Geometry: final body of the model. Coordinates: model frame, mm. Face numbers are marked on the shaded views. A direction names the side the tool comes from. Round coordinates to 2 decimals unless told otherwise and drop trailing zeros. Order: outer loops, then holes, each group sorted by start corner. A loop starts at its lowest first (then second) coordinate and runs counter-clockwise, first axis right, second up. Notation, with made-up numbers: M -26,14 L 8,14 A20 cw 8,52 Z; hole C -30.75,49.5 d8. An arc over 180 degrees is marked long. Return JSON: item names as keys, results as strings. Group by question number.
Q1. Contact query for flat-ended pins moving along their axis: pin 1 (3 mm diameter, centred on x = -41, z = 4.5, fed in from +Y); pin 2 (1.3 mm diameter, centred on y = 27, z = 6, fed in from +X). Output: stop coordinate, or through.
Q2. Ray query, probe 1 along X at (y, z) = (28, 4.5); probe 2 along X at (y, z) = (35.5, 2); probe 3 along X at (y, z) = (26.75, 7.75). Return the intervals inside material, ascending.
Q3. Cut plane B-B on y = 32. Output: boundary loops of the cut face in (x, z).
Q4. Access query for the marked faces 5, 6 and 7. Directions: +Z, -Z, +X, -X, +Y, -Y. A direction counts if a zero-diameter tool reaches every point of the face in a straight line with its end or side. Return the directions, or none.
Q5. Cut plane A-A on z = 5. Output: boundary loops of the cut face in (x, y).
Q6. Cut plane C-C on y = 20.5. Output: boundary loops of the cut face in (x, z), and give its area (3 significant figures).
Q7. Mould query, pull axis X, two halves, no side actions, for the marked faces 1, 2, 3 and 4. Classes: released by +X, released by -X, zero draft, split by the parting line, or undercut.
Q8. Cut plane D-D on x = -45. Output: boundary loops of the cut face in (y, z).
```python
from build123d import *

# Parameters (mm, degrees)
F0_W     = 20
F0_H     = 14.121413
F1_DEPTH = 10
F2_R     = 2.65
F3_DEPTH = 9.901
F5_DEPTH = 10


with BuildPart() as f1:
    # F0 (on Top) → F1 (new body)
    with BuildSketch(Plane.XY):
        with Locations((-41.761377, 22.08462)):
            Rectangle(F0_W, F0_H)
        with BuildLine():
            ThreePointArc((-25.361377, 20.023914), (-26.738101, 21.169687), (-25.861377, 22.731583))
            Line((-25.861377, 22.731583), (-25.861377, 26.782085))
            Line((-25.861377, 26.782085), (-25.861377, 27.804352))
            Line((-25.861377, 27.804352), (-25.861377, 36.782085))
            Line((-25.861377, 36.782085), (-28.861377, 36.782085))
            Line((-28.861377, 36.782085), (-28.861377, 29.145327))
            Line((-28.861377, 29.145327), (-31.761377, 29.145327))
            Line((-31.761377, 29.145327), (-31.761377, 15.023914))
            Line((-31.761377, 15.023914), (-25.361377, 15.023914))
            Line((-25.361377, 15.023914), (-25.361377, 20.023914))
        make_face()
        with BuildLine():
            ThreePointArc((-24.861377, 22.731583), (-23.984653, 21.169687), (-25.361377, 20.023914))
            Line((-25.361377, 20.023914), (-25.361377, 15.023914))
            ThreePointArc((-25.361377, 15.023914), (-19.227361, 19.59803), (-21.861377, 26.782085))
            Line((-21.861377, 26.782085), (-21.861377, 36.782085))
            Line((-21.861377, 36.782085), (-24.861377, 36.782085))
            Line((-24.861377, 36.782085), (-24.861377, 27.804352))
            Line((-24.861377, 27.804352), (-24.861377, 26.782085))
            Line((-24.861377, 26.782085), (-24.861377, 22.731583))
        make_face()
    extrude(amount=F1_DEPTH)

    # F2 (on face) → F3 (cut, through all)
    with BuildSketch(Plane(origin=(-28.861377, 0, 0), x_dir=(0, -1, 0), z_dir=(-1, 0, 0))):
        with Locations((-32.963706, 5)):
            Circle(F2_R)
    extrude(amount=-F3_DEPTH, mode=Mode.SUBTRACT)

    # F4 (on face) → F5 (cut)
    with BuildSketch(Plane(origin=(-28.861377, 0, 0), x_dir=(0, -1, 0), z_dir=(-1, 0, 0))):
        Polygon((-39.463706, 8.752777), (-39.463706, 1.247223), (-32.963706, -2.505553), (-26.463706, 1.247223), (-26.463706, 8.752777), (-32.963706, 12.505553), align=None)
    extrude(amount=F5_DEPTH, mode=Mode.SUBTRACT)


solid = f1.part
```
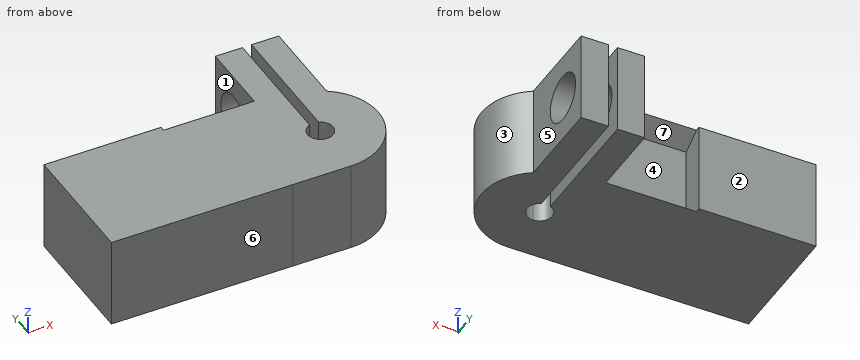
Result sheet:
{
 "1": {"pin 1": "stops at y = 29.15", "pin 2": "stops at x = -21.28"},
 "2": {"probe 1": "x = -51.76 to -38.86, -28.86 to -25.86, -24.86 to -21.86", "probe 2": "x = -28.86 to -25.86, -24.86 to -21.86", "probe 3": "x = -51.76 to -38.86, -28.86 to -25.86, -24.86 to -21.81"},
 "3": {"outline": "M -28.86,0 L -25.86,0 L -25.86,2.53 L -28.86,2.53 Z; M -28.86,7.47 L -25.86,7.47 L -25.86,10 L -28.86,10 Z; M -24.86,0 L -21.86,0 L -21.86,2.53 L -24.86,2.53 Z; M -24.86,7.47 L -21.86,7.47 L -21.86,10 L -24.86,10 Z"},
 "4": {"face 5": "+Z, -Z, +X, +Y", "face 6": "+Z, -Z, +X, -X, -Y", "face 7": "+Y"},
 "5": {"outline": "M -51.76,15.02 L -25.36,15.02 A6.4 ccw -21.86,26.78 L -21.86,30.31 L -24.86,30.31 L -24.86,22.73 A1.4 cw long -25.86,22.73 L -25.86,30.31 L -28.86,30.31 L -28.86,26.46 L -38.86,26.46 L -38.86,29.15 L -51.76,29.15 Z; M -28.86,35.61 L -25.86,35.61 L -25.86,36.78 L -28.86,36.78 Z; M -24.86,35.61 L -21.86,35.61 L -21.86,36.78 L -24.86,36.78 Z"},
 "6": {"outline": "M -51.76,0 L -26.41,0 L -26.41,10 L -51.76,10 Z; M -24.31,0 L -19.03,0 L -19.03,10 L -24.31,10 Z", "area": "306 mm²"},
 "7": {"face 1": "undercut", "face 2": "zero draft", "face 3": "released by +X", "face 4": "undercut"},
 "8": {"outline": "M 15.02,0 L 29.15,0 L 29.15,10 L 15.02,10 Z"}
}
